Solid Edge part; units mm, degrees
sketch "Sketch1" plane through (0, 0, 0) normal (0, 0, 1) x (1, 0, 0)
  line L0 (-60, 6.5) -> (-40, 6.5)
  line L1 (-40, 6.5) -> (-40, 12.5)
  line L2 (-40, 12.5) -> (-60, 12.5)
  line L3 (-60, 12.5) -> (-60, 6.5)
  line L4 (90, 6.5) -> (110, 6.5)
  line L5 (110, 6.5) -> (110, 12.5)
  line L6 (110, 12.5) -> (90, 12.5)
  line L7 (90, 12.5) -> (90, 6.5)
  line L8 (150, -37.5) -> (150, -22.5)
  line L9 (150, -22.5) -> (156, -22.5)
  line L10 (156, -22.5) -> (156, -2.5)
  line L11 (156, -2.5) -> (150, -2.5)
  line L12 (150, -2.5) -> (150, 37.5)
  line L13 (150, 37.5) -> (-100, 37.5)
  line L14 (-100, 37.5) -> (-100, -2.5)
  line L15 (-106, -2.5) -> (-100, -2.5)
  line L16 (-106, -22.5) -> (-106, -2.5)
  line L17 (-100, -22.5) -> (-106, -22.5)
  line L18 (-100, -22.5) -> (-100, -37.5)
  line L19 (-100, -37.5) -> (150, -37.5)
  dimension "D1" = 156
  dimension "D2" = 106
  dimension "D3" = 156
  dimension "D4" = 40
  dimension "D5" = 40
  dimension "D6" = 110
  dimension "D7" = 110
  dimension "D8" = 150
  dimension "D9" = 150
  dimension "D10" = 100
extrude "Protrusion1" add sketch "Sketch1" along normal blind 6
sketch "Sketch2" plane through (25, 0, 6) normal (0, 0, 1) x (1, 0, 0)
  line L0 (95, -2.5) -> (115, -2.5)
  line L1 (115, -2.5) -> (115, 0.5)
  line L2 (115, 0.5) -> (95, 0.5)
  line L3 (95, 0.5) -> (95, -2.5)
  dimension "D1" = 95
  dimension "D2" = 115
extrude "Cutout1" cut sketch "Sketch2" against normal through all
Model file for the job. Use its own axes, mm. A direction names the side the tool comes from. Give positions to 0.01 mm unless a question says otherwise; leave off trailing zeros. Loops run counter-clockwise (first coordinate to the right, second up) from the corner with the lowest first, then second, coordinate; pieces in that order, holes last.
1) Saw through at A-A (x = 126.5). Write the cut outline in (y, z).
2) Saw through at C-C (y = -28). Write the cut outline in (x, z).
3) Tool access for faces 5 (the flat face through (-103, -22.5, 3)), 6 (the flat face through (-100, 18, 3)), 7 (the flat face through (153, -22.5, 3)), 8 (the flat face through (110, 9, 3)): list every direction of +Z, -Z, +X, -X, +Y, -Y with a clear straight run to the whole face (end or side of a thin tool).
4) Saw through at B-B (z = 2.5). Write the cut outline in (x, y).
5) Flat gauge pins, fed straight in: pin 1 Ø3 at (x, z) = (-104.5, 2.5) entering from -Y; pin 2 Ø1.8 at (y, z) = (23, 2) entering from +X; pin 3 Ø3 at (y, z) = (8.5, 2.5) entering from -X; pin 4 Ø10 at (x, y) = (122.5, -27) entering from -Z. Where does each tip first touch, or does it go through?
6) Wall check: line 1 (X direction, y = 12, z = 0.3); line 2 (Y direction, x = -53, z = 1.85); line 3 (X direction, y = -25, z = 0.8). Give the ranges that are in metal, low to high.
7) Pull direction Y, two halves, no side cores. Call faces 1 (the flat face through (-100, -30, 3)), 2 (the flat face through (-103, -2.5, 3)), 3 (the flat face through (-40, 9, 3)), 4 (the flat face through (130, -2.5, 3)): +Y half, -Y half, draft (parallel to the pull), parting line (faces both ways), or undercut.
Answer block:
1. outline: (-37.5, 0) - (-2.5, 0) - (-2.5, 6) - (-37.5, 6) - close; (0.5, 0) - (37.5, 0) - (37.5, 6) - (0.5, 6) - close
2. outline: (-100, 0) - (150, 0) - (150, 6) - (-100, 6) - close
3. face 5: +Z, -Z, -X, -Y
3. face 6: +Z, -Z, -X, +Y
3. face 7: +Z, -Z, +X, -Y
3. face 8: +Z, -Z
4. outline: (-106, -22.5) - (-100, -22.5) - (-100, -37.5) - (150, -37.5) - (150, -22.5) - (156, -22.5) - (156, -2.5) - (150, -2.5) - (150, 37.5) - (-100, 37.5) - (-100, -2.5) - (-106, -2.5) - close; hole (-60, 6.5) - (-40, 6.5) - (-40, 12.5) - (-60, 12.5) - close; hole (90, 6.5) - (110, 6.5) - (110, 12.5) - (90, 12.5) - close; hole (120, -2.5) - (140, -2.5) - (140, 0.5) - (120, 0.5) - close
5. pin 1: stops at y = -22.5
5. pin 2: stops at x = 150
5. pin 3: stops at x = -100
5. pin 4: stops at z = 0
6. line 1: x = -100 to -60, -40 to 90, 110 to 150
6. line 2: y = -37.5 to 6.5, 12.5 to 37.5
6. line 3: x = -100 to 150
7. face 1: draft
7. face 2: +Y half
7. face 3: undercut
7. face 4: undercut
